CAD build for the part. Positions are in the model's coordinates, mm. Round coordinates to 2 decimals unless told otherwise and drop trailing zeros. Loops run counter-clockwise (first coordinate to the right, second up) from the corner with the lowest first, then second, coordinate; pieces in that order, holes last. Notation, with made-up numbers: M 35.5,-38.75 L 66.5,-38.75 A33 ccw 66.5,-9.75 Z; hole C 79,-32.75 d1. An arc over 180 degrees is marked long. One line per item, written item: value. Start each with the question number.
Autodesk Inventor part; units mm, degrees
ref_plane "YZ Plane" through (0, 0, 0) normal (1, 0, 0) x (0, 1, 0)
ref_plane "XZ Plane" through (0, 0, 0) normal (0, 1, 0) x (-1, 0, 0)
ref_plane "XY Plane" through (0, 0, 0) normal (0, 0, 1) x (1, 0, 0)
sketch "Sketch1" plane through (0, 0, 0) normal (0, 0, 1) x (1, 0, 0)
  line L0 (0, 0) -> (159, 0)
  line L1 (0, 0) -> (-100, 30)
  line L2 (0, 0) -> (236.9147, 0) construction
  line L3 (-100, 609.0812) -> (-100, 30)
  line L4 (90.9188, 800) -> (289, 800)
  line L5 (289, 800) -> (289, 560)
  line L6 (289, 560) -> (159, 560)
  line L7 (159, 235) -> (289, 235)
  line L8 (289, 325) -> (289, 235)
  line L9 (114, 203.5) -> (159, 203.5)
  line L10 (114, 228.5) -> (159, 228.5)
  arc A0 (114, 228.5) -> (114, 203.5) centre (114, 216) ccw
  line L11 (159, 0) -> (159, 203.5)
  line L12 (159, 228.5) -> (159, 235)
  line L13 (159, 560) -> (159, 325)
  line L14 (159, 325) -> (289, 325)
  line L15 (90.9188, 800) -> (-100, 609.0812)
  line L16 (90.9188, 800) -> (360.9188, 800) construction
  dimension "d0" = 159
  dimension "d3" = 100
  dimension "d6" = 800
  dimension "d7" = 240
  dimension "d8" = 130
  dimension "d11" = 235
  dimension "d14" = 25
  dimension "d16" = 216
  dimension "d18" = 45
  dimension "d19" = 389
  dimension "d22" = 130
  dimension "d23" = 235
  dimension "d25" = 30
  dimension "d26" = 270
  dimension "d27" = 135
extrude "Extrusion1" add sketch "Sketch1" along normal blind 1.6
fillet "Fillet1" radius 30 2 edges at (-100, 609.0812, 0.8) (90.9188, 800, 0.8)
equation "\"d22\" = d8"
equation "\"BendRadius\" = Thickness"
equation "\"BendReliefWidth\" = Thickness"
equation "\"BendReliefDepth\" = 0.5 * Thickness"
equation "\"CornerReliefSize\" = 4 * Thickness"
equation "\"MinimumRemnant\" = 2 * Thickness"
equation "\"TransitionRadius\" = BendRadius"
equation "\"JacobiRadiusSize\" = Thickness"
equation "\"GapSize\" = Thickness"
properties part number "Gearbox-Side Cover Part 1" material "Steel"
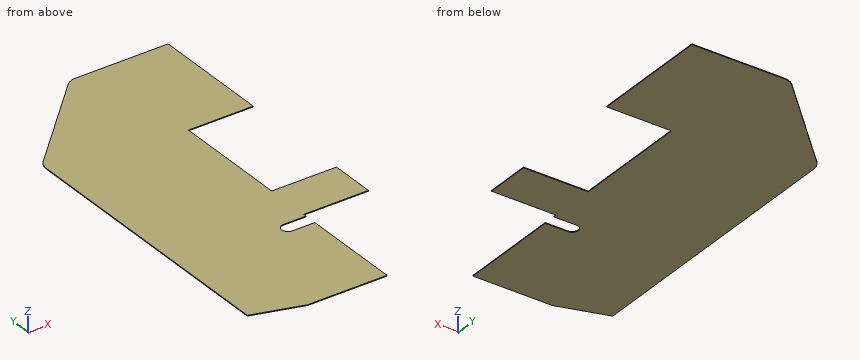
(1) Flat gauge pins, fed straight in: P1, Ø0.8, axis at y = 442.5, z = 0.5, coming from the +X side; P2, Ø0.5, axis at x = 223, z = 1, coming from the -Y side. Where does each tip first touch, or does it go through?
(2) Probe L1, parallel to Y at x = 263.5, z = 0.5; L2, parallel to Y at x = 141, z = 0.75; L3, parallel to X at y = 61.5, z = 0.45. List the from-to ranges inside material, lowest first.
(3) Slice it at B-B, the plane z = 1.15. List the corners of the cut face in (x, y).
(4) Slice it at D-D, the plane y = 486. List the corners of the cut face in (x, z).
(5) Slice it at A-A, the plane x = 145.5. List the corners of the cut face in (y, z).
(6) Slice it at C-C, the plane x = 224. List the corners of the cut face in (y, z).
Check result:
1. P1: stops at x = 159
1. P2: stops at y = 235
2. L1: y = 235 to 325, 560 to 800
2. L2: y = 0 to 203.5, 228.5 to 800
2. L3: x = -100 to 159
3. outline: M -100,30 L 0,0 L 159,0 L 159,203.5 L 114,203.5 A12.5 cw 114,228.5 L 159,228.5 L 159,235 L 289,235 L 289,325 L 159,325 L 159,560 L 289,560 L 289,800 L 103.35,800 A30 ccw 82.13,791.21 L -91.21,617.87 A30 ccw -100,596.65 Z
4. outline: M -100,0 L 159,0 L 159,1.6 L -100,1.6 Z
5. outline: M 0,0 L 203.5,0 L 203.5,1.6 L 0,1.6 Z; M 228.5,0 L 800,0 L 800,1.6 L 228.5,1.6 Z
6. outline: M 235,0 L 325,0 L 325,1.6 L 235,1.6 Z; M 560,0 L 800,0 L 800,1.6 L 560,1.6 Z
